Autodesk Inventor part; units mm, degrees
ref_plane "YZ Plane" through (0, 0, 0) normal (1, 0, 0) x (0, 1, 0)
ref_plane "XY Plane" through (0, 0, 0) normal (0, 0, 1) x (1, 0, 0)
sketch "Sketch1" plane through (0, 0, 0) normal (0, 0, 1) x (1, 0, 0)
  circle A0 centre (0, 0) radius 13.5
  circle A1 centre (0, 0) radius 16
  circle A2 centre (0, 0) radius 11
  dimension "d0" = 27
  dimension "d1" = 32
  dimension "d2" = 22
extrude "Extrusion1" add sketch "Sketch1" along normal blind 2.5 contours A0 | A1
extrude "Extrusion2" add sketch "Sketch1" against normal blind 7.5 contours A1
ref_plane "Work Plane1" through (0, -20, 0) normal (0, 1, 0) x (-1, 0, 0)
sketch "Sketch2" plane through (0, -20, 0) normal (0, 1, 0) x (-1, 0, 0)
  line L0 (-16, -7.5) -> (16, -7.5)
  line L1 (16, 2.5) -> (-16, 2.5)
  line L2 (16, -7.5) -> (16, 2.5)
  line L3 (-16, -7.5) -> (-16, 2.5)
  line L4 (-16, 2.5) -> (-26, 2.5)
  line L5 (-26, 2.5) -> (-26, -7.5)
  line L6 (-26, -7.5) -> (-16, -7.5)
  line L7 (-16, -7.5) -> (-16, 2.5)
  line L8 (16, 2.5) -> (26, 2.5)
  line L9 (26, 2.5) -> (26, -7.5)
  line L10 (26, -7.5) -> (16, -7.5)
  line L11 (16, -7.5) -> (16, 2.5)
  point P0 (0, 0)
  dimension "d8" = 10
  dimension "d9" = 10
  dimension "d10" = 10
  dimension "d11" = 10
extrude "Extrusion3" add sketch "Sketch2" along normal blind 20 contours L3 L1 L2 L0
delete faces "Delete Face1" heal yes whole lump no faces at (3.6667, 0, -5)
extrude "Extrusion4" add sketch "Sketch2" along normal blind 10 contours L6 L5 L4 L3 | L2 L8 L9 L10
properties part number "Adafruit_1528_4699_ND_House_02"
The listing builds one solid part. Answer for the finished solid, in the listing's coordinates (mm). A direction names the side the tool comes from. Round coordinates to 2 decimals unless told otherwise and drop trailing zeros. Loops run counter-clockwise (first coordinate to the right, second up) from the corner with the lowest first, then second, coordinate; pieces in that order, holes last.
1) For a pull along Y with two mould halves and no side action, classify faces 1 (the face through (0, -20, -2)), 2 (the face through (26, -15, -2)), 3 (the face through (-2.93, -13.18, -3.7)), 4 (the face through (-21, -10, -2)) as released by +Y, released by -Y, zero draft, split by the parting line, or undercut.
Outcome:
face 1: released by -Y
face 2: zero draft
face 3: undercut
face 4: released by +Y
2) Consider line 1 (Y direction, x = 0, z = -5.5); line 2 (X direction, y = 0, z = 1.05); line 3 (Y direction, x = 0, z = 1.85). Determine where each line is inside the solid, lowest interval first.
Outcome:
line 1: y = -20 to -13.5, 13.5 to 16
line 2: x = -16 to -11, 11 to 16
line 3: y = -20 to -11, 11 to 16
3) A cutting plane is placed at B-B on x = 0. Determine the outline of the cut face in (y, z), plus the area to 4 significant figures.
Outcome:
outline: (-20, -7.5) - (-13.5, -7.5) - (-13.5, 0) - (-11, 0) - (-11, 2.5) - (-20, 2.5) - close; (11, 0) - (13.5, 0) - (13.5, -7.5) - (16, -7.5) - (16, 2.5) - (11, 2.5) - close
area: 102.5 mm2
4) Given P1, Ø5, axis at y = -4.5, z = -4, coming from the -X side, flat-ended and moving along its own axis, determine where the tip first touches the part or whether it passes through.
Outcome:
P1: stops at x = -16
5) A cutting plane is placed at A-A on z = -6.25. Determine the outline of the cut face in (x, y).
Outcome:
outline: (-26, -20) - (26, -20) - (26, -10) - (16, -10) - (16, 0) arc R16 ccw to (-16, 0) - (-16, -10) - (-26, -10) - close; hole circle Ø27 at (0, 0)
6) For faces 5 (the face through (5, -10, 2.5)), 6 (the face through (-16, -5, -3)), 7 (the face through (4, -14, -7.5)), 8 (the face through (-5, -10, 0)), 9 (the face through (21, -10, -2)), determine the directions among +Z, -Z, +X, -X, +Y, -Y from which every point of the face is accessible in a straight line to the end or side of a thin tool.
Outcome:
face 5: +Z, +X, -X, +Y, -Y
face 6: +Z, -Z, -X, +Y
face 7: -Z, +X, -X, +Y, -Y
face 8: -Z
face 9: +Z, -Z, +X, +Y
7) A cutting plane is placed at C-C on y = 5.5. Determine the outline of the cut face in (x, z), plus the area to 3 significant figures.
Outcome:
outline: (-15.02, -7.5) - (-12.33, -7.5) - (-12.33, 0) - (-9.53, 0) - (-9.53, 2.5) - (-15.02, 2.5) - close; (9.53, 0) - (12.33, 0) - (12.33, -7.5) - (15.02, -7.5) - (15.02, 2.5) - (9.53, 2.5) - close
area: 67.9 mm2
